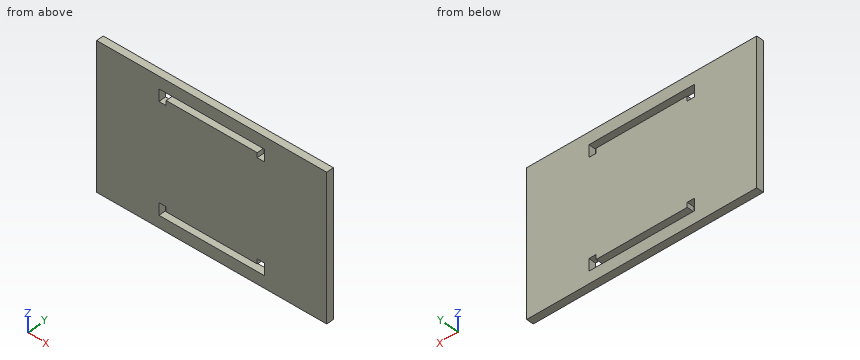
from build123d import *

# Parameters (mm, degrees)
SKETCH1_W           = 44
SKETCH1_H           = 5
BOSS_EXTRUDE1_DEPTH = 3


with BuildPart() as part:
    # Sketch1 → Boss-Extrude1 (new body)
    with BuildSketch(Plane(origin=(0, 0, 0), x_dir=(1, 0, 0), z_dir=(0, 1, 0))):
        with Locations((0, 27.5)):
            Rectangle(SKETCH1_W, SKETCH1_H)
        with Locations((0, -27.5)):
            Rectangle(SKETCH1_W, SKETCH1_H)
        Polygon((-22, -30), (-48, -30), (-48, 30), (-22, 30), (-22, 20), (-19, 20), (-19, 22), (19, 22), (19, 20), (22, 20), (22, 30), (48, 30), (48, -30), (22, -30), (22, -20), (19, -20), (19, -22), (-19, -22), (-19, -20), (-22, -20), align=None)
    extrude(amount=BOSS_EXTRUDE1_DEPTH)


solid = part.part
Read the model definition and answer for the solid it produces. Units are mm, in the model's axes. Coordinates: 2 decimals unless noted, no trailing zeros. Loops run counter-clockwise (first coordinate to the right, second up) from the corner with the lowest first, then second, coordinate; pieces in that order, holes last. Notation, with made-up numbers: (41, -5.5) -> (71, -5.5) arc R30 cw to (71, 23.5) -> close; hole circle Ø11 at (80, 49.5). An arc over 180 degrees is marked (long way). Write item = value, one per line. Start each with the question number.
1) Find the intervals of material crossed by L1, parallel to Z at x = -8, y = 1.9; L2, parallel to X at y = 1.6, z = -20.5; L3, parallel to X at y = 2.65, z = -23, in increasing order. Write a range as from..to.
2) The part is cut by section C-C, the plane y = 2.25. Determine the outline of the cut face in (x, z), plus the area to 3 significant figures.
3) The part is cut by section A-A, the plane x = 15. Determine the outline of the cut face in (y, z), plus the area to 3 significant figures.
4) The part is cut by section B-B, the plane z = -23. Determine the outline of the cut face in (x, y), plus the area to 3 significant figures.
Result:
q1.L1 = -30..-25, -22..22, 25..30
q1.L2 = -48..-22, -19..19, 22..48
q1.L3 = -48..-22, 22..48
q2.outline = (-48, -30) -> (48, -30) -> (48, 30) -> (-48, 30) -> close; hole (-22, -25) -> (22, -25) -> (22, -20) -> (19, -20) -> (19, -22) -> (-19, -22) -> (-19, -20) -> (-22, -20) -> close; hole (-22, 20) -> (-19, 20) -> (-19, 22) -> (19, 22) -> (19, 20) -> (22, 20) -> (22, 25) -> (-22, 25) -> close
q2.area = 5,470 mm²
q3.outline = (0, -30) -> (3, -30) -> (3, -25) -> (0, -25) -> close; (0, -22) -> (3, -22) -> (3, 22) -> (0, 22) -> close; (0, 25) -> (3, 25) -> (3, 30) -> (0, 30) -> close
q3.area = 162 mm²
q4.outline = (-48, 0) -> (-22, 0) -> (-22, 3) -> (-48, 3) -> close; (22, 0) -> (48, 0) -> (48, 3) -> (22, 3) -> close
q4.area = 156 mm²
